from build123d import *

# Parameters (mm, degrees)
SKETCH1_W           = 120
SKETCH1_H           = 90
BOSS_EXTRUDE1_DEPTH = 2
SKETCH2_R           = 4
SKETCH2_R_2         = 2
BOSS_EXTRUDE2_DEPTH = 4
FILLET1_R           = 5
BOSS_EXTRUDE3_DEPTH = 3
SKETCH4_R           = 4.5
CUT_EXTRUDE1_DEPTH  = 2
SKETCH5_R           = 4
SKETCH5_R_2         = 2.6
BOSS_EXTRUDE4_DEPTH = 2
SKETCH6_R           = 2.6
CUT_EXTRUDE2_DEPTH  = 163.360709533
CUT_EXTRUDE3_START  = -6.7
SKETCH7_R           = 2
CUT_EXTRUDE3_DEPTH  = 6.7


with BuildPart() as part:
    # Sketch1 → Boss-Extrude1 (new body)
    with BuildSketch(Plane(origin=(0, 0, 0), x_dir=(1, 0, 0), z_dir=(0, 1, 0))):
        with Locations((60, 45)):
            Rectangle(SKETCH1_W, SKETCH1_H)
    extrude(amount=BOSS_EXTRUDE1_DEPTH)

    # Sketch2 → Boss-Extrude2 (add)
    # profile 1 of 4: a face of its own
    with BuildSketch(Plane(origin=(0, 2, 0), x_dir=(1, 0, 0), z_dir=(0, 1, 0))):
        with Locations(Location((9.225, 83.15, 0), (0, 0, 90))):
            Circle(SKETCH2_R)
        with Locations(Location((9.225, 83.15, 0), (0, 0, 270))):
            Circle(SKETCH2_R_2, mode=Mode.SUBTRACT)
    # profile 2 of 4: a face of its own
    with BuildSketch(Plane(origin=(0, 2, 0), x_dir=(1, 0, 0), z_dir=(0, 1, 0))):
        with Locations(Location((9.225, 6.85, 0), (0, 0, 90))):
            Circle(SKETCH2_R)
        with Locations(Location((9.225, 6.85, 0), (0, 0, 270))):
            Circle(SKETCH2_R_2, mode=Mode.SUBTRACT)
    # profile 3 of 4: a face of its own
    with BuildSketch(Plane(origin=(0, 2, 0), x_dir=(1, 0, 0), z_dir=(0, 1, 0))):
        with Locations(Location((110.775, 83.15, 0), (0, 0, 90))):
            Circle(SKETCH2_R)
        with Locations(Location((110.775, 83.15, 0), (0, 0, 270))):
            Circle(SKETCH2_R_2, mode=Mode.SUBTRACT)
    # profile 4 of 4: a face of its own
    with BuildSketch(Plane(origin=(0, 2, 0), x_dir=(1, 0, 0), z_dir=(0, 1, 0))):
        with Locations(Location((110.775, 6.85, 0), (0, 0, 90))):
            Circle(SKETCH2_R)
        with Locations(Location((110.775, 6.85, 0), (0, 0, 270))):
            Circle(SKETCH2_R_2, mode=Mode.SUBTRACT)
    extrude(amount=BOSS_EXTRUDE2_DEPTH)

    # Fillet1
    fillet1_edges = [part.edges().sort_by_distance(p)[0] for p in [
        (120, 1, 0),
        (0, 1, 0),
    ]]
    fillet(fillet1_edges, radius=FILLET1_R)

    # Sketch3 → Boss-Extrude3 (add)
    with BuildSketch(Plane.XZ):
        with BuildLine():
            Line((5, 0), (115, 0))
            ThreePointArc((115, 0), (129.142135624, -5.857864376), (135, -20))
            Line((135, -20), (135, -80))
            ThreePointArc((135, -80), (132.071067812, -87.071067812), (125, -90))
            Line((125, -90), (-5, -90))
            ThreePointArc((-5, -90), (-12.071067812, -87.071067812), (-15, -80))
            Line((-15, -80), (-15, -20))
            ThreePointArc((-15, -20), (-9.142135624, -5.857864376), (5, 0))
        make_face()
    extrude(amount=BOSS_EXTRUDE3_DEPTH)

    # Sketch4 → Cut-Extrude1 (cut)
    with BuildSketch(Plane.XZ.offset(3)):
        with Locations(Location((-7.5, -17.5, 0), (0, 0, 270))):
            Circle(SKETCH4_R)
        with Locations(Location((-7.5, -82.5, 0), (0, 0, 270))):
            Circle(SKETCH4_R)
        with Locations(Location((127.5, -17.5, 0), (0, 0, 270))):
            Circle(SKETCH4_R)
        with Locations(Location((127.5, -82.5, 0), (0, 0, 270))):
            Circle(SKETCH4_R)
    extrude(amount=-CUT_EXTRUDE1_DEPTH, mode=Mode.SUBTRACT)

    # Sketch5 → Boss-Extrude4 (add)
    # profile 1 of 4: a face of its own
    with BuildSketch(Plane(origin=(0, 0, 0), x_dir=(1, 0, 0), z_dir=(0, 1, 0))):
        with Locations(Location((-7.5, 17.5, 0), (0, 0, 270))):
            Circle(SKETCH5_R)
        with Locations(Location((-7.5, 17.5, 0), (0, 0, 270))):
            Circle(SKETCH5_R_2, mode=Mode.SUBTRACT)
    # profile 2 of 4: a face of its own
    with BuildSketch(Plane(origin=(0, 0, 0), x_dir=(1, 0, 0), z_dir=(0, 1, 0))):
        with Locations(Location((127.5, 17.5, 0), (0, 0, 270))):
            Circle(SKETCH5_R)
        with Locations(Location((127.5, 17.5, 0), (0, 0, 270))):
            Circle(SKETCH5_R_2, mode=Mode.SUBTRACT)
    # profile 3 of 4: a face of its own
    with BuildSketch(Plane(origin=(0, 0, 0), x_dir=(1, 0, 0), z_dir=(0, 1, 0))):
        with Locations(Location((127.5, 82.5, 0), (0, 0, 270))):
            Circle(SKETCH5_R)
        with Locations(Location((127.5, 82.5, 0), (0, 0, 270))):
            Circle(SKETCH5_R_2, mode=Mode.SUBTRACT)
    # profile 4 of 4: a face of its own
    with BuildSketch(Plane(origin=(0, 0, 0), x_dir=(1, 0, 0), z_dir=(0, 1, 0))):
        with Locations(Location((-7.5, 82.5, 0), (0, 0, 270))):
            Circle(SKETCH5_R)
        with Locations(Location((-7.5, 82.5, 0), (0, 0, 270))):
            Circle(SKETCH5_R_2, mode=Mode.SUBTRACT)
    extrude(amount=BOSS_EXTRUDE4_DEPTH)

    # Sketch6 → Cut-Extrude2 (cut, through all)
    with BuildSketch(Plane(origin=(0, 0, 0), x_dir=(1, 0, 0), z_dir=(0, 1, 0))):
        with Locations(Location((-7.5, 17.5, 0), (0, 0, 90))):
            Circle(SKETCH6_R)
        with Locations(Location((127.5, 17.5, 0), (0, 0, 90))):
            Circle(SKETCH6_R)
        with Locations(Location((127.5, 82.5, 0), (0, 0, 90))):
            Circle(SKETCH6_R)
        with Locations(Location((-7.5, 82.5, 0), (0, 0, 90))):
            Circle(SKETCH6_R)
    extrude(amount=-CUT_EXTRUDE2_DEPTH, mode=Mode.SUBTRACT)

    # Sketch7 → Cut-Extrude3 (cut)
    with BuildSketch(Plane(origin=(0, 6, 0), x_dir=(1, 0, 0), z_dir=(0, 1, 0)).offset(CUT_EXTRUDE3_START)):
        with Locations(Location((110.775, 83.15, 0), (0, 0, 270))):
            Circle(SKETCH7_R)
        with Locations(Location((110.775, 6.85, 0), (0, 0, 270))):
            Circle(SKETCH7_R)
        with Locations(Location((9.225, 6.85, 0), (0, 0, 270))):
            Circle(SKETCH7_R)
        with Locations(Location((9.225, 83.15, 0), (0, 0, 270))):
            Circle(SKETCH7_R)
    extrude(amount=CUT_EXTRUDE3_DEPTH, mode=Mode.SUBTRACT)


solid = part.part
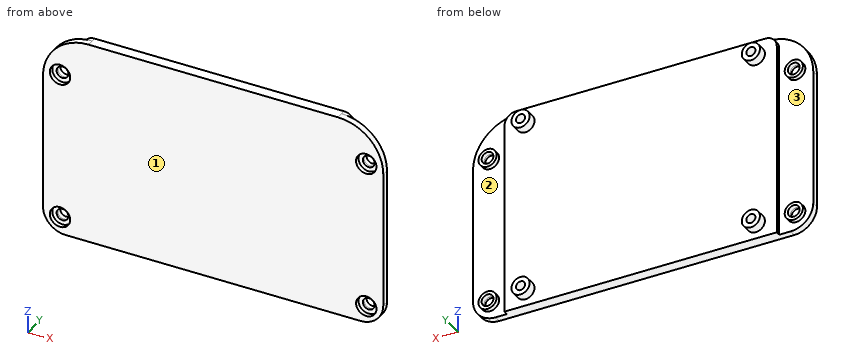
The listing builds one solid part. Answer for the finished solid, in the listing's coordinates (mm). Face numbers are marked on the shaded views. Coordinates: 2 decimals unless noted, no trailing zeros. Order: outer loops, then holes, each group sorted by start corner. A loop starts at its lowest first (then second) coordinate and runs counter-clockwise, first axis right, second up.
Q1. A cutting plane is placed at B-B, the plane z = -17.5. State how many separate pieces and enclosed holes the cut face has, and give its area (3 significant figures).
Q2. A cutting plane is placed at C-C, the plane x = -7.5. Write down the section's boundary in (y, z), and give its area (3 significant figures).
Q3. For a pull along Z with two mould halves and no side action, classify the marked faces 1, 2 and 3 as pulls with the +Z half, pulls with the -Z half, needs draft (parallel to the pull), parting line crosses it, or undercut.
Q4. Given P1, Ø2.5, axis at x = 126.5, z = -84, coming from the -Y side; P2, Ø3, axis at x = 100.5, y = 4, coming from the -Z side; P3, Ø3, axis at y = 2.5, z = -23.5, coming from the -X side; P4, Ø2, axis at x = 111, z = -82.5, coming from the +Y side, each flat-ended and moving along its own axis, determine where each tip first touches the part or whether it passes through.
Q5. Consider line 1 (X direction, y = 4.5, z = -8.5); line 2 (Z direction, x = 128.5, y = -1.25); line 3 (X direction, y = -0.4, z = -82.5). Determine where each line is inside the solid, lowest interval first.
Q6. A cutting plane is placed at D-D, the plane z = -72. Write down the section's boundary in (x, y).
Q7. A cutting plane is placed at A-A, the plane y = 3.75. Write down the section's boundary in (x, z) (3 decimals), and give its area (3 significant figures).
Answers follow:
1. separate pieces: 3
1. enclosed holes: 0
1. area: 654 mm2
2. outline: (-3, -89.68) - (0, -89.68) - (0, -86.5) - (2, -86.5) - (2, -85.1) - (-1, -85.1) - (-1, -87) - (-3, -87) - close; (-3, -78) - (-1, -78) - (-1, -79.9) - (2, -79.9) - (2, -78.5) - (0, -78.5) - (0, -21.5) - (2, -21.5) - (2, -20.1) - (-1, -20.1) - (-1, -22) - (-3, -22) - close; (-3, -13) - (-1, -13) - (-1, -14.9) - (2, -14.9) - (2, -13.5) - (0, -13.5) - (0, -4.39) - (-3, -4.39) - close
2. area: 221 mm2
3. face 1: needs draft
3. face 2: undercut
3. face 3: undercut
4. P1: stops at y = -1
4. P2: passes through
4. P3: stops at x = 0
4. P4: stops at y = -0.7
5. line 1: x = 5.58 to 8.09, 10.36 to 12.87, 107.13 to 109.64, 111.91 to 114.42
5. line 2: z = -89.37 to -86.89, -78.11 to -21.89, -13.11 to -5.24
5. line 3: x = -14.68 to -10.1, -4.9 to 7.33, 11.12 to 108.88, 112.67 to 124.9, 130.1 to 134.68
6. outline: (-15, -3) - (135, -3) - (135, 0) - (120, 0) - (120, 2) - (0, 2) - (0, 0) - (-15, 0) - close
7. outline: circle Ø8 at (9.225, -83.15); circle Ø8 at (9.225, -6.85); circle Ø8 at (110.775, -83.15); circle Ø8 at (110.775, -6.85); hole circle Ø4 at (9.225, -83.15); hole circle Ø4 at (9.225, -6.85); hole circle Ø4 at (110.775, -83.15); hole circle Ø4 at (110.775, -6.85)
7. area: 151 mm2
